Part model, mm, in its own coordinate system. A direction names the side the tool comes from. Round coordinates to 2 decimals unless told otherwise and drop trailing zeros. Order: outer loops, then holes, each group sorted by start corner. A loop starts at its lowest first (then second) coordinate and runs counter-clockwise, first axis right, second up. Notation, with made-up numbers: (11, 43.5) - (47, 43.5) arc R15 cw to (47, 50.5) - close; hole circle Ø1 at (-24, 19). An arc over 180 degrees is marked (long way). Return JSON: item names as keys, results as strings. Group by question number.
Item 1: Saw through at D-D on x = -0.5. List the corners of the cut face in (y, z).
Item 2: Probe probe 1 along Y at (x, z) = (-3, -7.7); probe 2 along X at (y, z) = (-0.4, -3); probe 3 along Y at (x, z) = (-3, -7.8). List the from-to ranges inside material, lowest first.
Item 3: Two-plate mould, pull along Z, no slides. Class faces 1 (the face through (7.43, -8.08, 7.4)), 2 (the face through (-3, -11, -7)), 3 (the face through (7, -4, -4)), 4 (the face through (0, 0, 0)): released by +Z, released by -Z, zero draft, split by the parting line, or undercut.
Item 4: Tool access for faces 5 (the face through (7, -12, 4)), 6 (the face through (3, -1, 3)), 7 (the face through (-3, -5, 7)), 8 (the face through (0.08, -0.6, 7.43)), 9 (the face through (-3, -15, -3)): list every direction of +Z, -Z, +X, -X, +Y, -Y with a clear straight run to the whole face (end or side of a thin tool).
Item 5: Saw through at B-B on z = -4.5. List the corners of the cut face in (x, y), and give its area (3 significant figures).
Item 6: Saw through at A-A on y = -8. List the corners of the cut face in (x, z).
Item 7: Drop flat-ended pins along their axis: pin 1 (2 mm diameter, centred on x = -3, z = -3, fed in from +Y); pin 2 (1.8 mm diameter, centred on x = -2.5, y = -11, fed in from -Z); pin 3 (2 mm diameter, centred on y = -11.75, z = 3.75, fed in from +X). Give the stop position or say it passes through.
```python
from build123d import *

# Parameters (mm, degrees)
F0_W      = 16
F0_H      = 16
F1_DEPTH  = 16
F2_R      = 2
F4_DEPTH  = 1
F5_R      = 1.75
F6_DEPTH  = 1
F8_DEPTH  = 1
F10_DEPTH = 1
F11_R     = 1.75
F12_DEPTH = 1
F14_DEPTH = 1


with BuildPart() as f1:
    # F0 (on Front) → F1 (new body)
    with BuildSketch(Plane.XZ):
        Rectangle(F0_W, F0_H)
    extrude(amount=F1_DEPTH)

    # F2
    f2_edges = [f1.edges().sort_by_distance(p)[0] for p in [
        (0, -16, 8),
        (-8, -8, 8),
        (8, -8, 8),
        (0, 0, 8),
        (0, 0, -8),
        (8, 0, 0),
        (-8, -8, -8),
        (-8, -16, 0),
        (-8, 0, 0),
        (0, -16, -8),
        (8, -16, 0),
        (8, -8, -8),
    ]]
    fillet(f2_edges, radius=F2_R)

    # F3 (on face) → F4 (cut)
    with BuildSketch(Plane.XZ.offset(16)):
        with BuildLine():
            Line((3, 1.25), (3, 3))
            Line((3, 3), (1.25, 3))
            ThreePointArc((1.25, 3), (1.7625631329, 1.7625631329), (3, 1.25))
        make_face()
        with BuildLine():
            Line((-3, -3), (-3, -1.25))
            ThreePointArc((-3, -1.25), (-4.2374368671, -4.2374368671), (-1.25, -3))
            Line((-1.25, -3), (-3, -3))
        make_face()
        with BuildLine():
            ThreePointArc((-1.25, -3), (-1.7625631329, -1.7625631329), (-3, -1.25))
            Line((-3, -1.25), (-3, -3))
            Line((-3, -3), (-1.25, -3))
        make_face()
        with BuildLine():
            Line((1.25, 3), (3, 3))
            Line((3, 3), (3, 1.25))
            ThreePointArc((3, 1.25), (4.2374368671, 1.7625631329), (4.75, 3))
            ThreePointArc((4.75, 3), (3, 4.75), (1.25, 3))
        make_face()
    extrude(amount=-F4_DEPTH, mode=Mode.SUBTRACT)

    # F5 (on face) → F6 (cut)
    with BuildSketch(Plane.XY.offset(8)):
        with BuildLine():
            Line((-3, -5), (-1.25, -5))
            ThreePointArc((-1.25, -5), (-4.2374368671, -3.7625631329), (-3, -6.75))
            Line((-3, -6.75), (-3, -5))
        make_face()
        with BuildLine():
            ThreePointArc((-3, -6.75), (-1.7625631329, -6.2374368671), (-1.25, -5))
            Line((-1.25, -5), (-3, -5))
            Line((-3, -5), (-3, -6.75))
        make_face()
        with BuildLine():
            Line((3, -11), (3, -9.25))
            ThreePointArc((3, -9.25), (1.7625631329, -9.7625631329), (1.25, -11))
            Line((1.25, -11), (3, -11))
        make_face()
        with BuildLine():
            ThreePointArc((4.75, -11), (4.2374368671, -9.7625631329), (3, -9.25))
            Line((3, -9.25), (3, -11))
            Line((3, -11), (1.25, -11))
            ThreePointArc((1.25, -11), (3, -12.75), (4.75, -11))
        make_face()
        with Locations((0, -8)):
            Circle(F5_R)
    extrude(amount=-F6_DEPTH, mode=Mode.SUBTRACT)

    # F7 (on face) → F8 (cut)
    with BuildSketch(Plane.YZ.offset(8)):
        with BuildLine():
            Line((-4.25, 3.75), (-6, 3.75))
            ThreePointArc((-6, 3.75), (-5.4874368671, 2.5125631329), (-4.25, 2))
            Line((-4.25, 2), (-4.25, 3.75))
        make_face()
        with BuildLine():
            ThreePointArc((-2.5, 3.75), (-4.25, 5.5), (-6, 3.75))
            Line((-6, 3.75), (-4.25, 3.75))
            Line((-4.25, 3.75), (-4.25, 2))
            ThreePointArc((-4.25, 2), (-3.0125631329, 2.5125631329), (-2.5, 3.75))
        make_face()
        with BuildLine():
            Line((-11.75, 3.75), (-10, 3.75))
            ThreePointArc((-10, 3.75), (-12.9874368671, 4.9874368671), (-11.75, 2))
            Line((-11.75, 2), (-11.75, 3.75))
        make_face()
        with BuildLine():
            ThreePointArc((-11.75, 2), (-10.5125631329, 2.5125631329), (-10, 3.75))
            Line((-10, 3.75), (-11.75, 3.75))
            Line((-11.75, 3.75), (-11.75, 2))
        make_face()
        with BuildLine():
            Line((-4.25, -3.75), (-4.25, -2))
            ThreePointArc((-4.25, -2), (-5.4874368671, -2.5125631329), (-6, -3.75))
            Line((-6, -3.75), (-4.25, -3.75))
        make_face()
        with BuildLine():
            ThreePointArc((-2.5, -3.75), (-3.0125631329, -2.5125631329), (-4.25, -2))
            Line((-4.25, -2), (-4.25, -3.75))
            Line((-4.25, -3.75), (-6, -3.75))
            ThreePointArc((-6, -3.75), (-4.25, -5.5), (-2.5, -3.75))
        make_face()
        with BuildLine():
            ThreePointArc((-10, -3.75), (-10.5125631329, -2.5125631329), (-11.75, -2))
            Line((-11.75, -2), (-11.75, -3.75))
            Line((-11.75, -3.75), (-10, -3.75))
        make_face()
        with BuildLine():
            Line((-11.75, -3.75), (-11.75, -2))
            ThreePointArc((-11.75, -2), (-12.9874368671, -4.9874368671), (-10, -3.75))
            Line((-10, -3.75), (-11.75, -3.75))
        make_face()
        with BuildLine():
            Line((-4.25, -1.75), (-4.25, 1.75))
            ThreePointArc((-4.25, 1.75), (-6, 0), (-4.25, -1.75))
        make_face()
        with BuildLine():
            ThreePointArc((-2.5, 0), (-3.0125631329, 1.2374368671), (-4.25, 1.75))
            Line((-4.25, 1.75), (-4.25, -1.75))
            ThreePointArc((-4.25, -1.75), (-3.0125631329, -1.2374368671), (-2.5, 0))
        make_face()
        with BuildLine():
            Line((-11.75, -1.75), (-11.75, 1.75))
            ThreePointArc((-11.75, 1.75), (-13.5, 0), (-11.75, -1.75))
        make_face()
        with BuildLine():
            ThreePointArc((-10, 0), (-10.5125631329, 1.2374368671), (-11.75, 1.75))
            Line((-11.75, 1.75), (-11.75, -1.75))
            ThreePointArc((-11.75, -1.75), (-10.5125631329, -1.2374368671), (-10, 0))
        make_face()
    extrude(amount=-F8_DEPTH, mode=Mode.SUBTRACT)

    # F9 (on face) → F10 (cut)
    with BuildSketch(Plane(origin=(0, 0, -8), x_dir=(1, 0, 0), z_dir=(0, 0, -1))):
        with BuildLine():
            Line((3, 11), (1.25, 11))
            ThreePointArc((1.25, 11), (1.7625631329, 9.7625631329), (3, 9.25))
            Line((3, 9.25), (3, 11))
        make_face()
        with BuildLine():
            ThreePointArc((4.75, 11), (3, 12.75), (1.25, 11))
            Line((1.25, 11), (3, 11))
            Line((3, 11), (3, 9.25))
            ThreePointArc((3, 9.25), (4.2374368671, 9.7625631329), (4.75, 11))
        make_face()
        with BuildLine():
            Line((-3, 11), (-1.25, 11))
            ThreePointArc((-1.25, 11), (-4.2374368671, 12.2374368671), (-3, 9.25))
            Line((-3, 9.25), (-3, 11))
        make_face()
        with BuildLine():
            ThreePointArc((-3, 9.25), (-1.7625631329, 9.7625631329), (-1.25, 11))
            Line((-1.25, 11), (-3, 11))
            Line((-3, 11), (-3, 9.25))
        make_face()
        with BuildLine():
            Line((3, 5), (3, 6.75))
            ThreePointArc((3, 6.75), (1.7625631329, 6.2374368671), (1.25, 5))
            Line((1.25, 5), (3, 5))
        make_face()
        with BuildLine():
            ThreePointArc((4.75, 5), (4.2374368671, 6.2374368671), (3, 6.75))
            Line((3, 6.75), (3, 5))
            Line((3, 5), (1.25, 5))
            ThreePointArc((1.25, 5), (3, 3.25), (4.75, 5))
        make_face()
        with BuildLine():
            ThreePointArc((-1.25, 5), (-1.7625631329, 6.2374368671), (-3, 6.75))
            Line((-3, 6.75), (-3, 5))
            Line((-3, 5), (-1.25, 5))
        make_face()
        with BuildLine():
            Line((-3, 5), (-3, 6.75))
            ThreePointArc((-3, 6.75), (-4.2374368671, 3.7625631329), (-1.25, 5))
            Line((-1.25, 5), (-3, 5))
        make_face()
    extrude(amount=-F10_DEPTH, mode=Mode.SUBTRACT)

    # F11 (on face) → F12 (cut)
    with BuildSketch(Plane(origin=(-8, 0, 0), x_dir=(0, -1, 0), z_dir=(-1, 0, 0))):
        with Locations((8, 0)):
            Circle(F11_R)
    extrude(amount=-F12_DEPTH, mode=Mode.SUBTRACT)

    # F13 (on face) → F14 (cut)
    with BuildSketch(Plane(origin=(0, 0, 0), x_dir=(-1, 0, 0), z_dir=(0, 1, 0))):
        with BuildLine():
            Line((3, 3), (1.25, 3))
            ThreePointArc((1.25, 3), (1.7625631329, 1.7625631329), (3, 1.25))
            Line((3, 1.25), (3, 3))
        make_face()
        with BuildLine():
            ThreePointArc((4.75, 3), (3, 4.75), (1.25, 3))
            Line((1.25, 3), (3, 3))
            Line((3, 3), (3, 1.25))
            ThreePointArc((3, 1.25), (4.2374368671, 1.7625631329), (4.75, 3))
        make_face()
        with BuildLine():
            Line((-3, 3), (-1.25, 3))
            ThreePointArc((-1.25, 3), (-4.2374368671, 4.2374368671), (-3, 1.25))
            Line((-3, 1.25), (-3, 3))
        make_face()
        with BuildLine():
            ThreePointArc((-3, 1.25), (-1.7625631329, 1.7625631329), (-1.25, 3))
            Line((-1.25, 3), (-3, 3))
            Line((-3, 3), (-3, 1.25))
        make_face()
        with BuildLine():
            Line((3, -3), (3, -1.25))
            ThreePointArc((3, -1.25), (1.7625631329, -1.7625631329), (1.25, -3))
            Line((1.25, -3), (3, -3))
        make_face()
        with BuildLine():
            ThreePointArc((4.75, -3), (4.2374368671, -1.7625631329), (3, -1.25))
            Line((3, -1.25), (3, -3))
            Line((3, -3), (1.25, -3))
            ThreePointArc((1.25, -3), (3, -4.75), (4.75, -3))
        make_face()
        with BuildLine():
            ThreePointArc((-1.25, -3), (-1.7625631329, -1.7625631329), (-3, -1.25))
            Line((-3, -1.25), (-3, -3))
            Line((-3, -3), (-1.25, -3))
        make_face()
        with BuildLine():
            Line((-3, -3), (-3, -1.25))
            ThreePointArc((-3, -1.25), (-4.2374368671, -4.2374368671), (-1.25, -3))
            Line((-1.25, -3), (-3, -3))
        make_face()
    extrude(amount=-F14_DEPTH, mode=Mode.SUBTRACT)


solid = f1.part
```
Filled in:
{
 "1": {"outline": "(-16, -6) arc R2 ccw to (-14, -8) - (-2, -8) arc R2 ccw to (0, -6) - (0, 6) arc R2 ccw to (-2, 8) - (-6.32, 8) - (-6.32, 7) - (-9.68, 7) - (-9.68, 8) - (-14, 8) arc R2 ccw to (-16, 6) - close"},
 "2": {"probe 1": "y = -15.05 to -12.75, -9.25 to -6.75, -3.25 to -0.95", "probe 2": "x = -7.2 to -4.75, -1.25 to 1.25, 4.75 to 7.2", "probe 3": "y = -14.87 to -12.75, -9.25 to -6.75, -3.25 to -1.13"},
 "3": {"face 1": "released by +Z", "face 2": "released by -Z", "face 3": "undercut", "face 4": "zero draft"},
 "4": {"face 5": "+X", "face 6": "+Y", "face 7": "+Z", "face 8": "+Z, +X, -X, +Y", "face 9": "-Y"},
 "5": {"outline": "(-8, -14) arc R2 ccw to (-6, -16) - (-3.9, -16) - (-3.9, -15) - (-2.1, -15) - (-2.1, -16) - (6, -16) arc R2 ccw to (8, -14) - (8, -13.33) - (7, -13.33) - (7, -10.17) - (8, -10.17) - (8, -5.83) - (7, -5.83) - (7, -2.67) - (8, -2.67) - (8, -2) arc R2 ccw to (6, 0) - (3.9, 0) - (3.9, -1) - (2.1, -1) - (2.1, 0) - (-2.1, 0) - (-2.1, -1) - (-3.9, -1) - (-3.9, 0) - (-6, 0) arc R2 ccw to (-8, -2) - close", "area": "241 mm^2"},
 "6": {"outline": "(-8, -6) arc R2 ccw to (-6, -8) - (6, -8) arc R2 ccw to (8, -6) - (8, 6) arc R2 ccw to (6, 8) - (1.75, 8) - (1.75, 7) - (-1.75, 7) - (-1.75, 8) - (-6, 8) arc R2 ccw to (-8, 6) - (-8, 1.75) - (-7, 1.75) - (-7, -1.75) - (-8, -1.75) - close"},
 "7": {"pin 1": "stops at y = -1", "pin 2": "stops at z = -7", "pin 3": "stops at x = 7"}
}
